The drawing under review shows one solid part. Ordinate dimensions are in mm from its lowest x, y, z. A direction names the side the tool comes from. Give positions to 0.01 mm unless a question says otherwise; leave off trailing zeros. Write each loop counter-clockwise with the first axis right and the second up, starting at its lowest first coordinate (ties: lowest second). Pieces come first, ordered by that corner, then holes. Notation, with made-up numbers: M -39.75,73.25 L -24.75,73.25 A20 ccw -24.75,84.25 Z; hole C 31,33.25 d8. An arc over 180 degrees is marked long. Write each question's results on one line, items separated by ' | '. Start each with the question number.
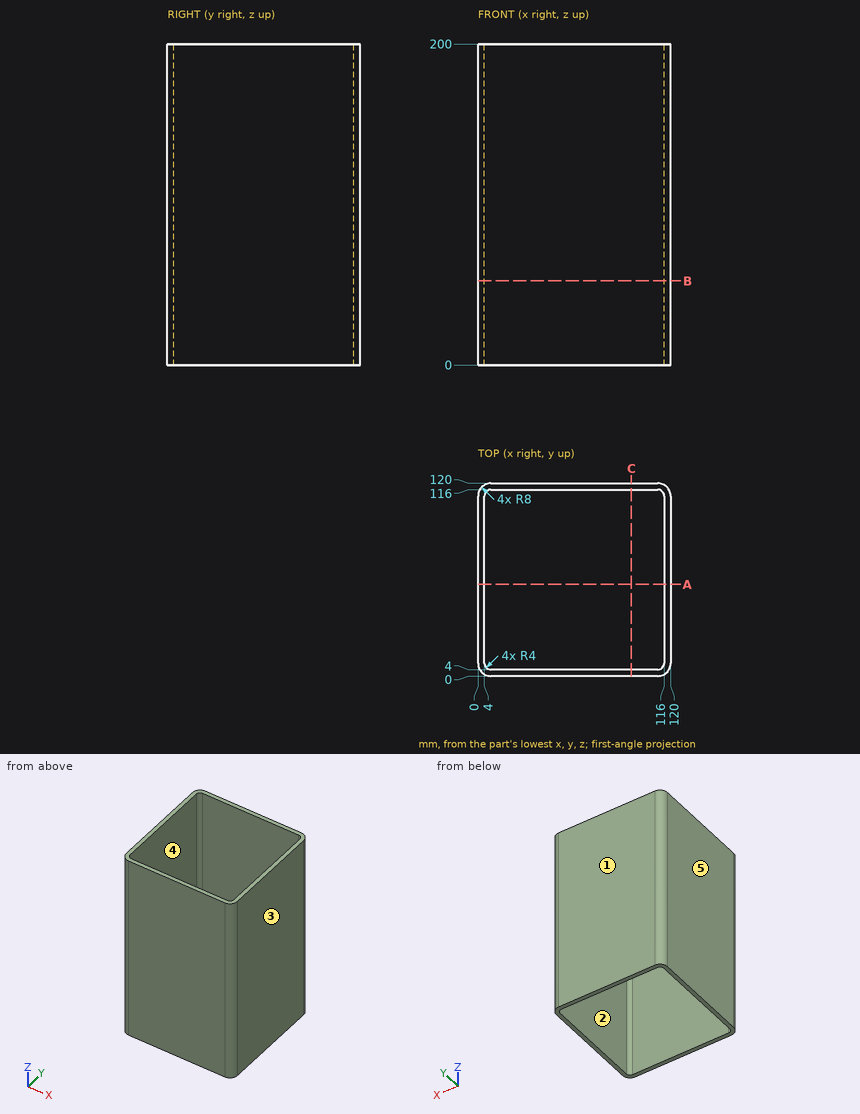
Q1. We need section B-B on z = 52.5. Write out the cut boundary in (x, y).
Q2. For the marked faces 1 and 2, list the 3-axis set-ups (+Z, -Z, +X, -X, +Y, -Y) from which the entire face can be reached by the end or side of a thin tool; tool diameter is ignored.
Q3. We need section A-A on y = 57. Write out the cut boundary in (x, z).
Q4. Wall thickness on line 1 along Y through (x, z) = (10, 69.5); line 2 along Y through (x, z) = (115.5, 20): over which ranges is each line inside the solid? List them lowest first. Write a range as from..to.
Q5. The part is to be moulded in two halves that separate along X. For the marked faces 3, 4 and 5, say which applies: pulls with the +X half, pulls with the -X half, needs draft (parallel to the pull), parting line crosses it, or undercut.
Answer sheet:
1) outline: M 0,8 A8 ccw 8,0 L 112,0 A8 ccw 120,8 L 120,112 A8 ccw 112,120 L 8,120 A8 ccw 0,112 Z; hole M 4,8 A4 ccw 8,4 L 112,4 A4 ccw 116,8 L 116,112 A4 ccw 112,116 L 8,116 A4 ccw 4,112 Z
2) face 1: +Z, -Z, +X, -X, +Y | face 2: +Z, -Z
3) outline: M 0,0 L 4,0 L 4,200 L 0,200 Z; M 116,0 L 120,0 L 120,200 L 116,200 Z
4) line 1: 0..4, 116..120 | line 2: 0.81..6.06, 113.94..119.19
5) face 3: pulls with the +X half | face 4: undercut | face 5: pulls with the -X half
